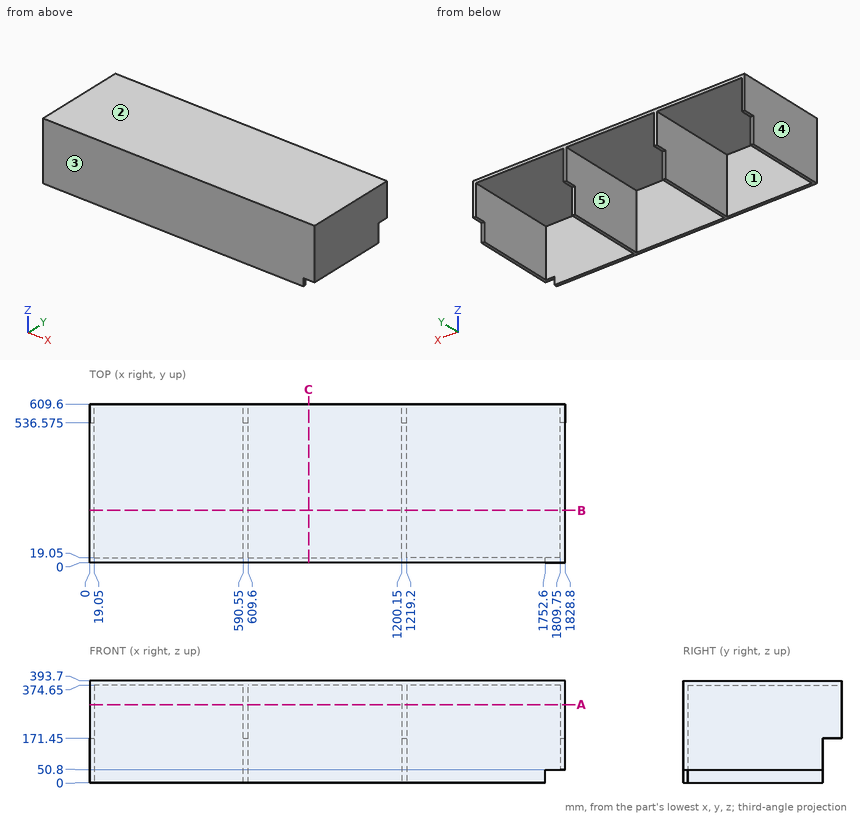
Verification items for this drawing (mm, ordinates from the low corner). A direction names the side the tool comes from. Round coordinates to 2 decimals unless told otherwise and drop trailing zeros. Order: outer loops, then holes, each group sorted by start corner. A loop starts at its lowest first (then second) coordinate and runs counter-clockwise, first axis right, second up. Notation, with made-up numbers: M 70.5,18 L 93.5,18 A19 ccw 93.5,52 Z; hole C 24,49.25 d10. An arc over 180 degrees is marked long. Answer in a Markdown table with one row per item. Add a question column.
Item 1: Sectioned sample at C-C, the plane x = 843. Enter the section's corners in (y, z).
Item 2: Sectioned sample at B-B, the plane y = 200. Enter the section's corners in (x, z), plus the area to 3 significant figures.
Item 3: Draft check along X on the marked faces 3, 4 and 5. Enter one of: released by +X, released by -X, zero draft, split by the parting line, or undercut.
Item 4: Set-up check for the marked faces 1 and 2: record each of +Z, -Z, +X, -X, +Y, -Y from which the full face is reachable in a straight line by a thin tool's end or side.
Item 5: Material ranges on L1, parallel to X at y = 127.5, z = 26; L2, parallel to X at y = 451, z = 348; L3, parallel to Y at x = 528, z = 258.5, recorded low to high. Write a range as [from, to].
Item 6: Depth check by flat-ended pin: pin 1 Ø8 at (x, z) = (457, 312.5) entering from +Y; pin 2 Ø21 at (x, z) = (8, 77.5) entering from +Y (3 decimals); pin 3 Ø21 at (y, z) = (9.5, 31) entering from +X. Enter the tip coordinate at first touch or a pass-through.
Item 7: Sectioned sample at A-A, the plane z = 300.5. Enter the section's corners in (x, y), plus the area to 3 significant figures.
Filled in:
| question | item | result |
|---|---|---|
| 1 | outline | M 0,0 L 19.05,0 L 19.05,374.65 L 609.6,374.65 L 609.6,393.7 L 0,393.7 Z |
| 2 | outline | M 0,0 L 19.05,0 L 19.05,374.65 L 590.55,374.65 L 590.55,0 L 609.6,0 L 609.6,374.65 L 1200.15,374.65 L 1200.15,0 L 1219.2,0 L 1219.2,374.65 L 1809.75,374.65 L 1809.75,50.8 L 1828.8,50.8 L 1828.8,393.7 L 0,393.7 Z |
| 2 | area | 62,400 mm² |
| 3 | face 3 | zero draft |
| 3 | face 4 | released by -X |
| 3 | face 5 | undercut |
| 4 | face 1 | -Z, +Y |
| 4 | face 2 | +Z, +X, -X, +Y, -Y |
| 5 | L1 | x = [0, 19.05], [590.55, 609.6], [1200.15, 1219.2] |
| 5 | L2 | x = [0, 19.05], [590.55, 609.6], [1200.15, 1219.2], [1809.75, 1828.8] |
| 5 | L3 | y = [0, 19.05] |
| 6 | pin 1 | stops at y = 19.05 |
| 6 | pin 2 | stops at y = 536.575 |
| 6 | pin 3 | stops at x = 1752.6 |
| 7 | outline | M 0,0 L 1828.8,0 L 1828.8,609.6 L 1809.75,609.6 L 1809.75,19.05 L 1219.2,19.05 L 1219.2,609.6 L 1200.15,609.6 L 1200.15,19.05 L 609.6,19.05 L 609.6,609.6 L 590.55,609.6 L 590.55,19.05 L 19.05,19.05 L 19.05,609.6 L 0,609.6 Z |
| 7 | area | 79,800 mm² |
